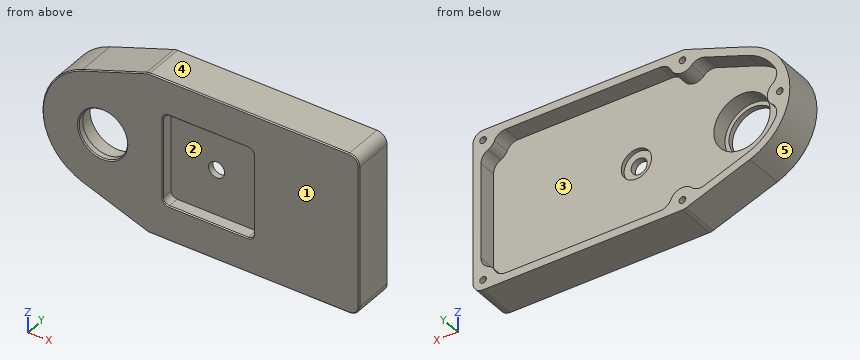
from build123d import *

# Parameters (mm, degrees)
SKETCH2_R                   = 4
SKETCH2_R_2                 = 12
BOSS_EXTRUDE1_DEPTH         = 20
FILLET1_R                   = 5
SKETCH2_3_R                 = 4
CUT_EXTRUDE1_DEPTH          = 6
SKETCH3_R                   = 14
CUT_EXTRUDE2_DEPTH          = 17
SKETCH4_R                   = 7.5
CUT_EXTRUDE3_DEPTH          = 11
TAP_DRILL_FOR_M4_TAP1_D     = 3.3
TAP_DRILL_FOR_M4_TAP1_DEPTH = 13
TAP_DRILL_FOR_M4_TAP1_TIP   = 0.991420021
CUT_EXTRUDE4_DEPTH          = 9
FILLET2_R                   = 6
CHAMFER1_SIZE               = 0.5


with BuildPart() as part:
    # Sketch2 → Boss-Extrude1 (new body)
    with BuildSketch(Plane(origin=(0, 0, 0), x_dir=(1, 0, 0), z_dir=(0, 1, 0))):
        with BuildLine():
            Line((-30, 40), (75, 40))
            Line((75, 40), (75, -40))
            Line((75, -40), (-30, -40))
            Line((-30, -40), (-62.673213991, -28.22243287))
            ThreePointArc((-62.673213991, -28.22243287), (-82.5, 0), (-62.673213991, 28.22243287))
            Line((-62.673213991, 28.22243287), (-30, 40))
        make_face()
        Circle(SKETCH2_R, mode=Mode.SUBTRACT)
        with Locations((-52.5, 0)):
            Circle(SKETCH2_R_2, mode=Mode.SUBTRACT)
    extrude(amount=BOSS_EXTRUDE1_DEPTH)

    # Fillet1
    fillet1_edges = [part.edges().sort_by_distance(p)[0] for p in [
        (-30, 10, -40),
        (75, 10, -40),
        (75, 10, 40),
        (-30, 10, 40),
    ]]
    fillet(fillet1_edges, radius=FILLET1_R)

    # Sketch2<3> → Cut-Extrude1 (cut)
    with BuildSketch(Plane(origin=(0, 0, 0), x_dir=(1, 0, 0), z_dir=(0, 1, 0))):
        with BuildLine():
            Line((22.6, -19.6), (22.6, 19.6))
            ThreePointArc((22.6, 19.6), (21.721320344, 21.721320344), (19.6, 22.6))
            Line((19.6, 22.6), (-19.6, 22.6))
            ThreePointArc((-19.6, 22.6), (-21.721320344, 21.721320344), (-22.6, 19.6))
            Line((-22.6, 19.6), (-22.6, -19.6))
            ThreePointArc((-22.6, -19.6), (-21.721320344, -21.721320344), (-19.6, -22.6))
            Line((-19.6, -22.6), (19.6, -22.6))
            ThreePointArc((19.6, -22.6), (21.721320344, -21.721320344), (22.6, -19.6))
        make_face()
        Circle(SKETCH2_3_R, mode=Mode.SUBTRACT)
    extrude(amount=CUT_EXTRUDE1_DEPTH, mode=Mode.SUBTRACT)

    # Sketch3 → Cut-Extrude2 (cut)
    with BuildSketch(Plane(origin=(0, 20, 0), x_dir=(1, 0, 0), z_dir=(0, 1, 0))):
        with Locations((-52.5, 0)):
            Circle(SKETCH3_R)
    extrude(amount=-CUT_EXTRUDE2_DEPTH, mode=Mode.SUBTRACT)

    # Sketch4 → Cut-Extrude3 (cut)
    with BuildSketch(Plane(origin=(0, 20, 0), x_dir=(1, 0, 0), z_dir=(0, 1, 0))):
        Circle(SKETCH4_R)
    extrude(amount=-CUT_EXTRUDE3_DEPTH, mode=Mode.SUBTRACT)

    # Tap Drill for M4 Tap1
    with Locations(Plane(origin=(0, 20, 0), x_dir=(1, 0, 0), z_dir=(0, 1, 0))):
        with Locations((70, 35), (-77.5, 0), (-29.126349288, 35), (-29.126349288, -35), (70, -35)):
            Hole(TAP_DRILL_FOR_M4_TAP1_D / 2, depth=TAP_DRILL_FOR_M4_TAP1_DEPTH)
            with Locations((0, 0, -(TAP_DRILL_FOR_M4_TAP1_DEPTH + TAP_DRILL_FOR_M4_TAP1_TIP / 2))):  # 118° drill point
                Cone(0, TAP_DRILL_FOR_M4_TAP1_D / 2, TAP_DRILL_FOR_M4_TAP1_TIP, mode=Mode.SUBTRACT)

    # Sketch7 → Cut-Extrude4 (cut)
    with BuildSketch(Plane(origin=(0, 20, 0), x_dir=(1, 0, 0), z_dir=(0, 1, 0))):
        with BuildLine():
            Line((-61.316785459, -24.459441821), (-35.269382186, -33.848632633))
            ThreePointArc((-35.269382186, -33.848632633), (-28.050584319, -28.843277679), (-22.956867948, -36))
            Line((-22.956867948, -36), (63.83051866, -36))
            ThreePointArc((63.83051866, -36), (65.580582618, -30.580582618), (71, -28.83051866))
            Line((71, -28.83051866), (71, 28.83051866))
            ThreePointArc((71, 28.83051866), (65.580582618, 30.580582618), (63.83051866, 36))
            Line((63.83051866, 36), (-22.956867948, 36))
            ThreePointArc((-22.956867948, 36), (-28.050584319, 28.843277679), (-35.269382186, 33.848632633))
            Line((-35.269382186, 33.848632633), (-61.316785459, 24.459441821))
            ThreePointArc((-61.316785459, 24.459441821), (-71.810161981, 17.410274101), (-77.73875, 6.24543821))
            ThreePointArc((-77.73875, 6.24543821), (-71.25, 0), (-77.73875, -6.24543821))
            ThreePointArc((-77.73875, -6.24543821), (-71.810161981, -17.410274101), (-61.316785459, -24.459441821))
        make_face()
    extrude(amount=-CUT_EXTRUDE4_DEPTH, mode=Mode.SUBTRACT)

    # Fillet2
    fillet2_edges = [part.edges().sort_by_distance(p)[0] for p in [
        (71, 15.5, 28.83051866),
        (63.83051866, 15.5, 36),
        (-22.956867948, 15.5, 36),
        (-35.269382186, 15.5, 33.848632633),
        (-77.73875, 15.5, 6.24543821),
        (-77.73875, 15.5, -6.24543821),
        (-35.269382186, 15.5, -33.848632633),
        (-22.956867948, 15.5, -36),
        (63.83051866, 15.5, -36),
        (71, 15.5, -28.83051866),
    ]]
    fillet(fillet2_edges, radius=FILLET2_R)

    # Chamfer1
    chamfer1_edges = [part.edges().sort_by_distance(p)[0] for p in [
        (-46.747549472, 0, 33.963085841),
        (-82.5, 0, 0),
        (-64.5, 0, 0),
        (20.436825356, 0, 40),
        (-46.747549472, 0, -33.963085841),
        (20.436825356, 0, -40),
        (75, 0, 0),
        (-29.986961262, 0, -39.925377856),
        (73.535533906, 0, -38.535533906),
        (73.535533906, 0, 38.535533906),
        (-29.986961262, 0, 39.925377856),
        (22.6, 0, 0),
        (21.721320344, 0, -21.721320344),
        (0, 0, -22.6),
        (-21.721320344, 0, -21.721320344),
        (21.721320344, 0, 21.721320344),
        (0, 0, 22.6),
        (-21.721320344, 0, 21.721320344),
        (-22.6, 0, 0),
    ]]
    chamfer(chamfer1_edges, length=CHAMFER1_SIZE)


solid = part.part
Input: part model. Units: mm. Frame: model coordinates. Face numbers are marked on the shaded views. A direction names the side the tool comes from. Round coordinates to 2 decimals unless told otherwise and drop trailing zeros. Order: outer loops, then holes, each group sorted by start corner. A loop starts at its lowest first (then second) coordinate and runs counter-clockwise, first axis right, second up. Notation, with made-up numbers: (9, 64.5) - (56, 64.5) arc R24 cw to (56, 75.5) - close; hole circle Ø9 at (-7.75, 56.5). An arc over 180 degrees is marked (long way). Use a Markdown table: item, result.
1. Section D-D on x = 51.5. Return the cut outline in (y, z), then the cut area to 3 significant figures.
Evaluation:
| item | result |
|---|---|
| outline | (0, -39.5) - (0.5, -40) - (20, -40) - (20, -36) - (11, -36) - (11, 36) - (20, 36) - (20, 40) - (0.5, 40) - (0, 39.5) - close |
| area | 952 mm^2 |
2. Material intervals for probe 1 along Z at (x, y) = (33, 13); probe 2 along X at (y, z) = (16.5, -1); probe 3 along Z at (x, y) = (70, 13), sorted ascending.
Evaluation:
| item | result |
|---|---|
| probe 1 | -40 to -36, 36 to 40 |
| probe 2 | -82.48 to -78.81, -76.19 to -71.33, 71 to 75 |
| probe 3 | -40 to -36.65, -33.35 to -27.13, 27.13 to 33.35, 36.65 to 40 |
3. Access query for the marked faces 1 and 2. Directions: +Z, -Z, +X, -X, +Y, -Y. A direction counts if a zero-diameter tool reaches every point of the face in a straight line with its end or side. Return the directions, or none.
Evaluation:
| item | result |
|---|---|
| face 1 | +Z, -Z, +X, -X, -Y |
| face 2 | -Y |
4. Section C-C on y = 18. State how many separate pieces and enclosed holes the cut face has, then the cut area to 3 significant figures.
Evaluation:
| item | result |
|---|---|
| separate pieces | 1 |
| enclosed holes | 6 |
| area | 1,960 mm^2 |
5. First-contact query: pin 1 (6 mm diameter, centred on y = 3, z = -8, fed in from -X); pin 2 (24 mm diameter, centred on x = 0, z = 0, fed in from -Y); pin 3 (21.5 mm diameter, centred on x = -2, z = 5, fed in from +Y). Flat tips, straight axial feed; report the tip coordinate or a pass-through.
Evaluation:
| item | result |
|---|---|
| pin 1 | x = -82.08 |
| pin 2 | y = 6 |
| pin 3 | y = 11 |
6. Section A-A on y = 4.5. Return the cut outline in (x, z), then the cut area to 3 significant figures.
Evaluation:
| item | result |
|---|---|
| outline | (-62.67, -28.22) - (-30.82, -39.7) arc R5 ccw to (-29.13, -40) - (70, -40) arc R5 ccw to (75, -35) - (75, 35) arc R5 ccw to (70, 40) - (-29.13, 40) arc R5 ccw to (-30.82, 39.7) - (-62.67, 28.22) arc R30 ccw to start; hole circle Ø28 at (-52.5, 0); hole (-22.6, -19.6) arc R3 ccw to (-19.6, -22.6) - (19.6, -22.6) arc R3 ccw to (22.6, -19.6) - (22.6, 19.6) arc R3 ccw to (19.6, 22.6) - (-19.6, 22.6) arc R3 ccw to (-22.6, 19.6) - close |
| area | 8,780 mm^2 |
7. Section B-B on x = 0. Return the cut outline in (y, z), then the cut area to 3 significant figures.
Evaluation:
| item | result |
|---|---|
| outline | (0, -39.5) - (0.5, -40) - (20, -40) - (20, -36) - (11, -36) - (11, -7.5) - (9, -7.5) - (9, -4) - (6, -4) - (6, -22.6) - (0.5, -22.6) - (0, -23.1) - close; (0, 23.1) - (0.5, 22.6) - (6, 22.6) - (6, 4) - (9, 4) - (9, 7.5) - (11, 7.5) - (11, 36) - (20, 36) - (20, 40) - (0.5, 40) - (0, 39.5) - close |
| area | 626 mm^2 |
8. Mould query, pull axis X, two halves, no side actions, for the marked faces 3, 4 and 5. Classes: +X half, -X half, draft (parallel to the pull), parting line (faces both ways), or undercut.
Evaluation:
| item | result |
|---|---|
| face 3 | undercut |
| face 4 | draft |
| face 5 | -X half |
